```python
from build123d import *

# Parameters (mm, degrees)
SKETCH1_W           = 215.9
SKETCH1_H           = 76.2
BOSS_EXTRUDE1_DEPTH = 6.35
BOSS_EXTRUDE2_DEPTH = 12.7
BOSS_EXTRUDE2_TAPER = 2
BOSS_EXTRUDE3_DEPTH = 3.175
SKETCH4_W           = 6.35
SKETCH4_H           = 6.35
CUT_EXTRUDE1_DEPTH  = 118.26027686


with BuildPart() as part:
    # Sketch1 → Boss-Extrude1 (new body)
    with BuildSketch(Plane(origin=(0, 0, 0), x_dir=(1, 0, 0), z_dir=(0, 1, 0))):
        Rectangle(SKETCH1_W, SKETCH1_H)
    extrude(amount=BOSS_EXTRUDE1_DEPTH)

    # Sketch2 → Boss-Extrude2 (add)
    with BuildSketch(Plane(origin=(0, 6.35, 0), x_dir=(1, 0, 0), z_dir=(0, 1, 0))):
        Polygon((-44.45, -38.1), (107.95, -38.1), (107.95, 38.1), (-44.45, 38.1), (-44.45, 25.4), (-42.8625, 25.4), (-42.8625, 36.5125), (106.3625, 36.5125), (106.3625, -36.5125), (-42.8625, -36.5125), (-42.8625, -25.4), (-44.45, -25.4), align=None)
    extrude(amount=BOSS_EXTRUDE2_DEPTH, taper=BOSS_EXTRUDE2_TAPER)

    # Sketch3 → Boss-Extrude3 (add, symmetric)
    with BuildSketch(Plane.XY):
        Polygon((-107.95, 6.35), (-107.95, 31.75), (-101.6, 31.75), (-98.425, 28.575), (-98.425, 25.4), (-104.775, 25.4), (-104.775, 6.35), align=None)
    extrude(amount=BOSS_EXTRUDE3_DEPTH, both=True)

    # Sketch4 → Cut-Extrude1 (cut, through all)
    with BuildSketch(Plane(origin=(0, 6.35, 0), x_dir=(1, 0, 0), z_dir=(0, 1, 0))):
        with Locations((-101.6, 0)):
            Rectangle(SKETCH4_W, SKETCH4_H)
    extrude(amount=-CUT_EXTRUDE1_DEPTH, mode=Mode.SUBTRACT)


solid = part.part
```
Can you work these out from the model? Positions are in its coordinate system, mm. A direction names the side the tool comes from. Give positions to 0.01 mm unless a question says otherwise; leave off trailing zeros. Loops run counter-clockwise (first coordinate to the right, second up) from the corner with the lowest first, then second, coordinate; pieces in that order, holes last. Notation, with made-up numbers: M -7,84 L 51,84 A28 cw 51,122 Z; hole C -17.5,46 d9. An arc over 180 degrees is marked long. Use CSV: the item, a comma, the result in double quotes. Start each with the question number.
1. On a 3-axis mill with a long thin cutter (end or side, diameter ignored), from which of +Z, -Z, +X, -X, +Y, -Y can I reach the whole of each face in a straight line? I mean faces 4 (the face through (-105, 22, -3.175)), 5 (the face through (-105, 22, 3.175)), 6 (the face through (-102, 3, 3.175)). Say none if no direction works.
2. Imagine slicing it at A-A, the plane x = -65. Write out the boundary of the cut face in (y, z).
3. If we mould it in two halves opening along X, with no side actions, what happens to faces 1 (the face through (-2, 3, 38.1)), 2 (the face through (-107.95, 8, 0)), 3 (the face through (-104.775, 13, 0))? For each: released by +X, released by -X, zero draft, split by the parting line, or undercut.
4. For P1, Ø1, axis at y = 10, z = -3, coming from the +X side; P2, Ø3, axis at y = 9.5, z = -1, coming from the +X side; P3, Ø23, axis at x = -41.5, z = 0, coming from the +Y side, each with a flat end and sliding along its axis, tell me the tip position at first contact or that it passes through.
5. If I drill on L1, parallel to X at y = 7, z = -27; L2, parallel to Z at x = -15, y = 7.5; L3, parallel to Z at x = -33, y = 7, over which ranges is the centre line in solid material (lowest first)?
Response values:
1,face 4,"-Z, -X, +Y"
1,face 5,"+Z, -X, +Y"
1,face 6,"-Y"
2,outline,"M 0,-38.1 L 6.35,-38.1 L 6.35,38.1 L 0,38.1 Z"
3,face 1,"zero draft"
3,face 2,"released by -X"
3,face 3,"undercut"
4,P1,"x = 107.84"
4,P2,"x = 107.89"
4,P3,"y = 6.35"
5,L1,"-44.43 to -42.89, 106.39 to 107.93"
5,L2,"-38.06 to -36.55, 36.55 to 38.06"
5,L3,"-38.08 to -36.54, 36.54 to 38.08"
